Autodesk Inventor part; units mm, degrees
ref_plane "YZ Plane" through (0, 0, 0) normal (1, 0, 0) x (0, 1, 0)
ref_plane "XZ Plane" through (0, 0, 0) normal (0, 1, 0) x (-1, 0, 0)
ref_plane "XY Plane" through (0, 0, 0) normal (0, 0, 1) x (1, 0, 0)
sketch "Sketch1" plane through (0, 0, 0) normal (0, 1, 0) x (-1, 0, 0)
  arc A0 (30.7371, -16.74) -> (16.74, -30.7371) centre (0, 0) ccw
  line L0 (30.7371, -16.74) -> (16.74, -30.7371)
  circle A1 centre (11.3137, 0) radius 1.5
  line L1 (0, -11.3137) -> (11.3137, 0) construction
  line L2 (11.3137, 0) -> (0, 11.3137) construction
  circle A2 centre (0, -11.3137) radius 1.5
  circle A3 centre (0, 11.3137) radius 1.5
  line L3 (0, 11.3137) -> (-11.3137, 0) construction
  line L4 (-11.3137, 0) -> (0, -11.3137) construction
  line L5 (11.3137, 0) -> (-11.3137, 0) construction
  line L6 (0, -11.3137) -> (0, 11.3137) construction
  circle A4 centre (-11.3137, 0) radius 1.5
  circle A5 centre (0, 0) radius 3
  dimension "d2" = 70
  dimension "d13" = 16
  dimension "d14" = 3
  dimension "d16" = 6
extrude "Extrusion1" add sketch "Sketch1" along normal blind 10
sketch "Sketch3" plane through (-30.7371, 0, -16.74) normal (-0.7071, 0, -0.7071) x (-0.7071, 0, 0.7071)
  line L0 (-19.7949, 0) -> (0, 0) construction
  line L1 (-19.7949, 10) -> (0, 10) construction
  line L2 (0, 0) -> (-19.7949, 10) construction
  circle A0 centre (-9.8974, 5) radius 1.5
  point P0 (-9.8974, 0)
  dimension "d17" = 3
extrude "Extrusion3" add sketch "Sketch3" along normal blind 5
properties part number "Pulley-35"
CAD build for the part. Positions are in the model's coordinates, mm. Round coordinates to 2 decimals unless told otherwise and drop trailing zeros. Order: outer loops, then holes, each group sorted by start corner. A loop starts at its lowest first (then second) coordinate and runs counter-clockwise, first axis right, second up. Notation, with made-up numbers: (60, 78) - (80, 78) arc R13 ccw to (80, 90) - close; hole circle Ø7 at (12.5, 34.25). An arc over 180 degrees is marked (long way). Answer in a Markdown table with one row per item. Add a question column.
(1) Probe L1, parallel to Z at x = 0, y = 4.5; L2, parallel to Z at x = -11.5, y = 9.75; L3, parallel to X at y = 4.5, z = -27. List the from-to ranges inside material, lowest first. Write a range as [from, to].
(2) Band-saw the part on D-D on z = -8. List the corners of the cut face in (x, y), and give its area (3 significant figures).
(3) Drop flat-ended pins along their axis: pin 1 Ø1.5 at (x, y) = (-13.5, 7) entering from -Z (3 decimals); pin 2 Ø4 at (x, y) = (-8.5, 6) entering from -Z; pin 3 Ø4 at (x, y) = (-19.5, 6) entering from -Z. Give the stop position or say it passes through.
(4) Band-saw the part on B-B on x = 0. List the corners of the cut face in (y, z).
(5) Band-saw the part on A-A on z = 0. List the corners of the cut face in (x, y), and give its area (3 significant figures).
(6) Mould opens along Z. For faces 1 (the face through (-24.42, 4.93, -26.54)), 2 (the face through (-27.26, 5.02, -27.29)), 3 (the face through (25.72, 4.93, 23.74)), 4 (the face through (0, 10, -7)) say: +Z half, -Z half, draft (parallel to the pull), parting line (faces both ways), or undercut.
(7) Band-saw the part on C-C on y = 8.5. List the corners of the cut face in (x, z), and give its area (3 significant figures).
Data:
| question | item | result |
|---|---|---|
| 1 | L1 | z = [-35, -12.81], [-9.81, -3], [3, 9.81], [12.81, 35] |
| 1 | L2 | z = [-33.06, -1.49], [1.49, 33.06] |
| 1 | L3 | x = [-27.55, -25], [-20.48, 22.27] |
| 2 | outline | (-34.07, 0) - (34.07, 0) - (34.07, 10) - (-34.07, 10) - close |
| 2 | area | 681 mm^2 |
| 3 | pin 1 | stops at z = -32.595 |
| 3 | pin 2 | stops at z = -34.39 |
| 3 | pin 3 | stops at z = -29.98 |
| 4 | outline | (0, -35) - (10, -35) - (10, -12.81) - (0, -12.81) - close; (0, -9.81) - (10, -9.81) - (10, -3) - (0, -3) - close; (0, 3) - (10, 3) - (10, 9.81) - (0, 9.81) - close; (0, 12.81) - (10, 12.81) - (10, 35) - (0, 35) - close |
| 5 | outline | (-35, 0) - (-12.81, 0) - (-12.81, 10) - (-35, 10) - close; (-9.81, 0) - (-3, 0) - (-3, 10) - (-9.81, 10) - close; (3, 0) - (9.81, 0) - (9.81, 10) - (3, 10) - close; (12.81, 0) - (35, 0) - (35, 10) - (12.81, 10) - close |
| 5 | area | 580 mm^2 |
| 6 | face 1 | undercut |
| 6 | face 2 | -Z half |
| 6 | face 3 | parting line |
| 6 | face 4 | draft |
| 7 | outline | (-30.74, -16.74) - (-16.74, -30.74) arc R35 ccw (long way) to start; hole circle Ø3 at (-11.31, 0); hole circle Ø6 at (0, 0); hole circle Ø3 at (0, -11.31); hole circle Ø3 at (0, 11.31); hole circle Ø3 at (11.31, 0) |
| 7 | area | 3,770 mm^2 |
